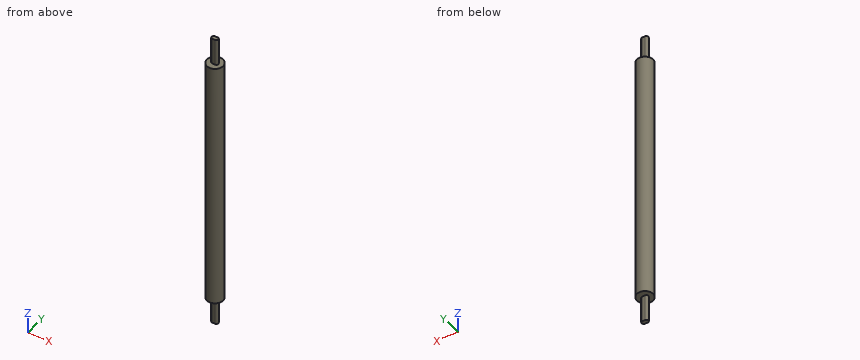
```python
from build123d import *

# Parameters (mm, degrees)
ESQUISSE1_R        = 6
BOSS_EXTRU_1_DEPTH = 190
BOSS_EXTRU_2_DEPTH = 20
BOSS_EXTRU_3_START = 20
BOSS_EXTRU_3_DEPTH = 20


with BuildPart() as part:
    # Esquisse1 → Boss.-Extru.1 (new body)
    with BuildSketch(Plane.XY):
        Circle(ESQUISSE1_R)
    extrude(amount=BOSS_EXTRU_1_DEPTH)

    # Esquisse2 → Boss.-Extru.2 (add)
    with BuildSketch(Plane.XY.offset(190)):
        with BuildLine():
            Line((-1, 1.5), (1, 1.5))
            ThreePointArc((1, 1.5), (2.5, 0), (1, -1.5))
            Line((1, -1.5), (-1, -1.5))
            ThreePointArc((-1, -1.5), (-2.5, 0), (-1, 1.5))
        make_face()
    extrude(amount=BOSS_EXTRU_2_DEPTH)

    # Esquisse3 → Boss.-Extru.3 (add)
    with BuildSketch(Plane(origin=(0, 0, 0), x_dir=(-1, 0, 0), z_dir=(0, 0, -1)).offset(BOSS_EXTRU_3_START)):
        with BuildLine():
            Line((-1, 1.5), (1, 1.5))
            ThreePointArc((1, 1.5), (2.5, 0), (1, -1.5))
            Line((1, -1.5), (-1, -1.5))
            ThreePointArc((-1, -1.5), (-2.5, 0), (-1, 1.5))
        make_face()
    extrude(amount=-BOSS_EXTRU_3_DEPTH)


solid = part.part
```
Can you work these out from the model? Positions are in its coordinate system, mm. Round coordinates to 2 decimals unless told otherwise and drop trailing zeros. Loops run counter-clockwise (first coordinate to the right, second up) from the corner with the lowest first, then second, coordinate; pieces in that order, holes last. Notation, with made-up numbers: M -23,81 L -9,81 A21 ccw -9,95 Z; hole C -35,19 d6. An arc over 180 degrees is marked long. Answer in a Markdown table with one row per item.
1. If we section it at A-A, the plane z = 136: Please give me the cut outline in (x, y), plus the area to 3 significant figures.
Established:
| item | result |
|---|---|
| outline | C 0,0 d12 |
| area | 113 mm² |
2. Please list where these lines run through material, in increasing order: line 1 (Z direction, x = 3.25, y = -3); line 2 (Y direction, x = -0.25, z = 128); line 3 (Y direction, x = -5.5, z = 87). Write a range as from..to.
Established:
| item | result |
|---|---|
| line 1 | 0..190 |
| line 2 | -5.99..5.99 |
| line 3 | -2.4..2.4 |
3. I'm going to push flat-ended pins straight in: pin 1 Ø1 at (x, z) = (0.5, -13) entering from -Y; pin 2 Ø3 at (x, y) = (-4.5, 2) entering from -Z; pin 3 Ø3 at (x, z) = (2, 60) entering from -Y. Where does each tip first touch, or does it pass through?
Established:
| item | result |
|---|---|
| pin 1 | y = -1.5 |
| pin 2 | z = 0 |
| pin 3 | y = -5.98 |
